```python
from build123d import *

# Parameters (mm, degrees)
SKETCH_R     = 1.15
SKETCH_W     = 108.5
SKETCH_H     = 43
PAD_DEPTH    = 4.6
FILLET_R     = 3
POCKET_DEPTH = 2.6


with BuildPart() as part:
    # Sketch → Pad (new body)
    with BuildSketch(Plane.XY):
        Polygon((-69.25, 56.5), (-79.25, 56.5), (-79.25, 46.5), (-59.25, 26.5), (-59.25, -26.5), (-79.25, -46.5), (-79.25, -56.5), (-69.25, -56.5), (-49.25, -36.5), (49.25, -36.5), (69.25, -56.5), (79.25, -56.5), (79.25, -46.5), (59.25, -26.5), (59.25, 26.5), (79.25, 46.5), (79.25, 56.5), (69.25, 56.5), (49.25, 36.5), (-49.25, 36.5), align=None)
        with Locations((-74.25, 51.5)):
            Circle(SKETCH_R, mode=Mode.SUBTRACT)
        with Locations((74.25, 51.5)):
            Circle(SKETCH_R, mode=Mode.SUBTRACT)
        with Locations((-74.25, -51.5)):
            Circle(SKETCH_R, mode=Mode.SUBTRACT)
        with Locations((74.25, -51.5)):
            Circle(SKETCH_R, mode=Mode.SUBTRACT)
        Rectangle(SKETCH_W, SKETCH_H, mode=Mode.SUBTRACT)
    extrude(amount=PAD_DEPTH)

    # Fillet
    fillet_edges = [part.edges().sort_by_distance(p)[0] for p in [
        (79.25, -56.5, 2.3),
        (79.25, 56.5, 2.3),
        (-79.25, 56.5, 2.3),
        (-79.25, -56.5, 2.3),
    ]]
    fillet(fillet_edges, radius=FILLET_R)

    # Sketch001 (on Face5 of Fillet) → Pocket (cut)
    with BuildSketch(Plane.XY.offset(4.6)):
        Polygon((-71.565321, 49.95), (-71.565321, 53.05), (-74.25, 54.6), (-76.934679, 53.05), (-76.934679, 49.95), (-74.25, 48.4), align=None)
        Polygon((-71.565321, -53.05), (-71.565321, -49.95), (-74.25, -48.4), (-76.934679, -49.95), (-76.934679, -53.05), (-74.25, -54.6), align=None)
        Polygon((76.934679, -53.05), (76.934679, -49.95), (74.25, -48.4), (71.565321, -49.95), (71.565321, -53.05), (74.25, -54.6), align=None)
        Polygon((76.934679, 49.95), (76.934679, 53.05), (74.25, 54.6), (71.565321, 53.05), (71.565321, 49.95), (74.25, 48.4), align=None)
    extrude(amount=-POCKET_DEPTH, mode=Mode.SUBTRACT)


solid = part.part
```
Build history of the part. All positions in model axes, mm. A direction names the side the tool comes from. Round coordinates to 2 decimals unless told otherwise and drop trailing zeros. Write each loop counter-clockwise with the first axis right and the second up, starting at its lowest first coordinate (ties: lowest second). Pieces come first, ordered by that corner, then holes.
1) 3-axis set-ups, long thin cutter, end or side, ignore diameter. For faces 1 (the flat face through (-1, -21.5, 2)), 2 (the flat face through (-69.11, -36.36, 2.27)), 3 (the flat face through (-59.39, -46.64, 2.27)), 4 (the flat face through (74, 50, 2)): which of +Z, -Z, +X, -X, +Y, -Y reach the whole face in a straight line?
2) Pin check, flat tips, straight feed: pin 1 (3.5 mm diameter, centred on x = 74.25, y = 51.5, fed in from +Z); pin 2 (2.5 mm diameter, centred on y = 6, z = 3, fed in from +X); pin 3 (1.5 mm diameter, centred on y = -19, z = 2, fed in from -X). Stop position of each tip, or through.
3) Drill centre lines: probe 1 along Y at (x, z) = (27, 1.75); probe 2 along X at (y, z) = (-14, 2.4); probe 3 along X at (y, z) = (-51.5, 1.5). Where is each one in solid material? Low to high.
4) Band-saw the part on B-B, the plane x = 24.5. List the corners of the cut face in (y, z), and give its area (3 significant figures).
5) Band-saw the part on A-A, the plane y = 5.5. List the corners of the cut face in (x, z), and give its area (3 significant figures).
6) Band-saw the part on C-C, the plane z = 0.7. Give the number of separate pieces and of enclosed holes in the cut face, and give its area (3 significant figures).
7) Mould opens along X. For faces 5 (the flat face through (79.25, -50, 2)), 6 (the flat face through (-79.25, -50, 2)), 7 (the flat face through (74, -53, 2)) say: +X half, -X half, draft (parallel to the pull), parting line (faces both ways), or undercut.
8) Band-saw the part on D-D, the plane y = 24.5. List the corners of the cut face in (x, z), and give its area (3 significant figures).
Ans:
1. face 1: +Z, -Z
1. face 2: +Z, -Z, -X
1. face 3: +Z, -Z, -Y
1. face 4: +Z
2. pin 1: stops at z = 2
2. pin 2: stops at x = 59.25
2. pin 3: stops at x = -59.25
3. probe 1: y = -36.5 to -21.5, 21.5 to 36.5
3. probe 2: x = -59.25 to -54.25, 54.25 to 59.25
3. probe 3: x = -79.25 to -75.4, -73.1 to -64.25, 64.25 to 73.1, 75.4 to 79.25
4. outline: (-36.5, 0) - (-21.5, 0) - (-21.5, 4.6) - (-36.5, 4.6) - close; (21.5, 0) - (36.5, 0) - (36.5, 4.6) - (21.5, 4.6) - close
4. area: 138 mm2
5. outline: (-59.25, 0) - (-54.25, 0) - (-54.25, 4.6) - (-59.25, 4.6) - close; (54.25, 0) - (59.25, 0) - (59.25, 4.6) - (54.25, 4.6) - close
5. area: 46.0 mm2
6. separate pieces: 1
6. enclosed holes: 5
6. area: 5,560 mm2
7. face 5: +X half
7. face 6: -X half
7. face 7: undercut
8. outline: (-59.25, 0) - (59.25, 0) - (59.25, 4.6) - (-59.25, 4.6) - close
8. area: 545 mm2
